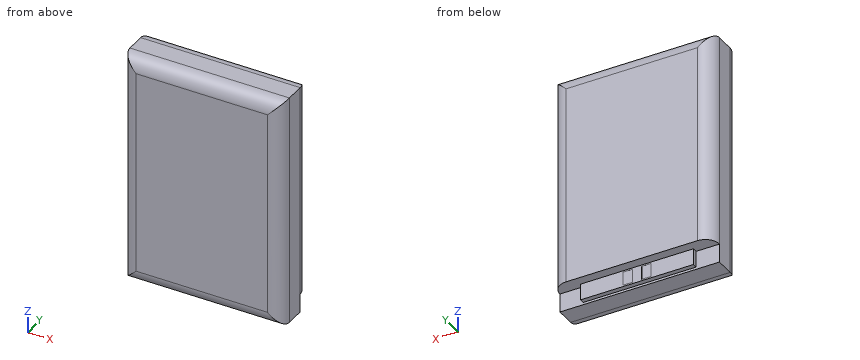
from build123d import *

# Parameters (mm, degrees)
SKETCH_1_W          = 34
SKETCH_1_H          = 50
EXTRUDE_1_DEPTH     = 10
FILLET_1_R          = 3
SKETCH_2_W          = 36
SKETCH_2_H          = 5
CUT_EXTRUDE_1_DEPTH = 3
SKETCH_3_W          = 24
SKETCH_3_H          = 3.5
EXTRUDE_2_DEPTH     = 1
SKETCH_4_W          = 2
SKETCH_4_H          = 2.9
CUT_EXTRUDE_2_DEPTH = 0.01


with BuildPart() as part:
    # Эскиз1 → Бобышка-Вытянуть1 (new body)
    with BuildSketch(Plane(origin=(0, 0, 0), x_dir=(1, 0, 0), z_dir=(0, 1, 0))):
        Rectangle(SKETCH_1_W, SKETCH_1_H)
    extrude(amount=EXTRUDE_1_DEPTH)

    # Скругление1
    fillet_1_edges = [part.edges().sort_by_distance(p)[0] for p in [
        (17, 10, 0),
        (-17, 10, 0),
        (0, 0, -25),
        (17, 0, 0),
        (0, 0, 25),
        (-17, 0, 0),
        (0, 10, 25),
    ]]
    fillet(fillet_1_edges, radius=FILLET_1_R)

    # Эскиз2 → Вырез-Вытянуть1 (cut)
    with BuildSketch(Plane(origin=(0, 10, 0), x_dir=(1, 0, 0), z_dir=(0, 1, 0))):
        with Locations((0, 23.5)):
            Rectangle(SKETCH_2_W, SKETCH_2_H)
    extrude(amount=-CUT_EXTRUDE_1_DEPTH, mode=Mode.SUBTRACT)

    # Эскиз3 → Бобышка-Вытянуть2 (add)
    with BuildSketch(Plane(origin=(0, 7, 0), x_dir=(1, 0, 0), z_dir=(0, 1, 0))):
        with Locations((0, 22.75)):
            Rectangle(SKETCH_3_W, SKETCH_3_H)
    extrude(amount=EXTRUDE_2_DEPTH)

    # Эскиз4 → Вырез-Вытянуть2 (cut)
    with BuildSketch(Plane(origin=(0, 8, 0), x_dir=(1, 0, 0), z_dir=(0, 1, 0))):
        with Locations((-2, 22.75)):
            Rectangle(SKETCH_4_W, SKETCH_4_H)
        with Locations((2, 22.75)):
            Rectangle(SKETCH_4_W, SKETCH_4_H)
    extrude(amount=-CUT_EXTRUDE_2_DEPTH, mode=Mode.SUBTRACT)


solid = part.part
Design review of the part built by this model. Coordinates are the model's own, in mm. Coordinates: 2 decimals unless noted, no trailing zeros. Loops run counter-clockwise (first coordinate to the right, second up) from the corner with the lowest first, then second, coordinate; pieces in that order, holes last. Notation, with made-up numbers: (16.25, -18.5) -> (21.25, -18.5) arc R18 ccw to (21.25, -7.5) -> close; hole circle Ø3 at (55.5, -14). An arc over 180 degrees is marked (long way). Use a Markdown table: item, result. Add a question column.
Item 1: We need section B-B, the plane z = 6.5. Write out the cut boundary in (x, y), and give its area (3 significant figures).
Item 2: We need section A-A, the plane x = 0.5. Write out the cut boundary in (y, z), and give its area (3 significant figures).
Item 3: Wall thickness on L1, parallel to Z at x = 3, y = 2.75; L2, parallel to Y at x = -10.5, z = -22; L3, parallel to X at y = 7.25, z = 21.5: over which ranges is each line inside the solid? List them lowest first. Write a range as from..to.
Item 4: Clearance check with flat-ended pins moving along their axes: P1, Ø2.5, axis at x = -3, y = 9, coming from the -Z side; P2, Ø3, axis at x = -5, z = -24, coming from the +Y side. State where each tip first meets the part, or that it passes through.
Item 5: We need section C-C, the plane y = 2. Write out the cut boundary in (x, z), and give its area (3 significant figures).
Numbers:
| question | item | result |
|---|---|---|
| 1 | outline | (-17, 3) arc R3 ccw to (-14, 0) -> (14, 0) arc R3 ccw to (17, 3) -> (17, 7) arc R3 ccw to (14, 10) -> (-14, 10) arc R3 ccw to (-17, 7) -> close |
| 1 | area | 332 mm^2 |
| 2 | outline | (0, -22) arc R3 ccw to (3, -25) -> (7, -25) -> (7, -24.5) -> (8, -24.5) -> (8, -21) -> (10, -21) -> (10, 22) arc R3 ccw to (7, 25) -> (3, 25) arc R3 ccw to (0, 22) -> close |
| 2 | area | 486 mm^2 |
| 3 | L1 | z = -24.99..24.99 |
| 3 | L2 | y = 0..8 |
| 3 | L3 | x = -16.99..16.99 |
| 4 | P1 | stops at z = -24.5 |
| 4 | P2 | stops at y = 8 |
| 5 | outline | (-16.83, -24.83) -> (16.83, -24.83) -> (16.83, 24.83) -> (-16.83, 24.83) -> close |
| 5 | area | 1,670 mm^2 |
